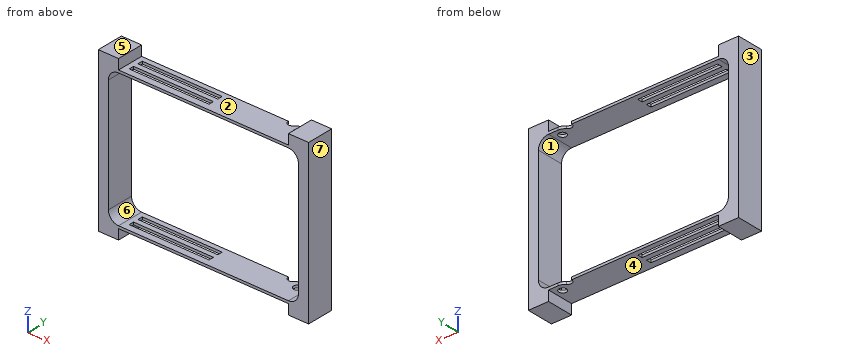
from build123d import *

# Parameters (mm, degrees)
F0_W      = 113
F0_H      = 80
F1_DEPTH  = 15.875
F2_R      = 6
F3_W      = 89
F3_H      = 3
F3_W_2    = 95
F3_R      = 1.5
F4_DEPTH  = 132
F5_W      = 42.9403819144
F5_H      = 7.4070980772
F6_DEPTH  = 1.5
F7_W      = 42.8083911538
F7_H      = 7.2430414148
F8_DEPTH  = 1.5
F9_R      = 2.5
F10_DEPTH = 92
F11_R     = 2.25
F12_DEPTH = 200
F13_R     = 5


with BuildPart() as f1:
    # F0 (on Front) → F1 (new body)
    with BuildSketch(Plane.XZ):
        Polygon((-50.5, 47.5), (-62.5, 47.5), (-62.5, -47.5), (-50.5, -47.5), (-50.5, -41.5), (50.5, -41.5), (50.5, -47.5), (62.5, -47.5), (62.5, 47.5), (50.5, 47.5), (50.5, 41.5), (-50.5, 41.5), align=None)
        Rectangle(F0_W, F0_H, mode=Mode.SUBTRACT)
    extrude(amount=F1_DEPTH)

    # F2
    f2_edges = [f1.edges().sort_by_distance(p)[0] for p in [
        (56.5, -7.9375, 40),
        (56.5, -7.9375, -40),
        (-56.5, -7.9375, -40),
        (-56.5, -7.9375, 40),
    ]]
    fillet(f2_edges, radius=F2_R)

    # F3 (on face) → F4 (cut)
    with BuildSketch(Plane.XY.offset(41.5)):
        with Locations((-3, -4.5)):
            Rectangle(F3_W, F3_H)
        with Locations((0, -10.5)):
            Rectangle(F3_W_2, F3_H)
        with Locations((46, -4.5)):
            Circle(F3_R)
    extrude(amount=-F4_DEPTH, mode=Mode.SUBTRACT)

    # F5 (on face) → F6 (join)
    with BuildSketch(Plane.XY.offset(41.5)):
        with Locations((21.4701909572, -3.7035490386)):
            Rectangle(F5_W, F5_H)
        Polygon((42.9403819144, -7.4070980772), (0, -7.4070980772), (0, -14.1382440925), (49.1435937583, -14.1382440925), (49.1435937583, -7.4070980772), align=None)
    extrude(amount=-F6_DEPTH)

    # F7 (on face) → F8 (join)
    with BuildSketch(Plane(origin=(0, 0, -41.5), x_dir=(1, 0, 0), z_dir=(0, 0, -1))):
        Polygon((49.0116067231, 15.875), (0, 15.875), (0, 7.2430414148), (42.8083911538, 7.2430414148), (49.0116067231, 7.2430414148), align=None)
        with Locations((21.4041955769, 3.6215207074)):
            Rectangle(F7_W, F7_H)
    extrude(amount=-F8_DEPTH)

    # F9 (on face) → F10 (cut)
    with BuildSketch(Plane.XY.offset(41.5)):
        with Locations((39.25, 0)):
            Circle(F9_R)
    extrude(amount=-F10_DEPTH, mode=Mode.SUBTRACT)

    # F11 (on face) → F12 (cut)
    with BuildSketch(Plane.XY.offset(41.5)):
        with Locations((46, -4.5)):
            Circle(F11_R)
    extrude(amount=-F12_DEPTH, mode=Mode.SUBTRACT)

    # F13
    f13_edges = [f1.edges().sort_by_distance(p)[0] for p in [
        (41.75, 0, 40.75),
        (41.75, 0, -40.75),
    ]]
    fillet(f13_edges, radius=F13_R)


solid = f1.part
The model under review builds one solid part; all positions refer to its coordinate system, in mm. Face numbers are marked on the shaded views. A direction names the side the tool comes from. Round coordinates to 2 decimals unless told otherwise and drop trailing zeros. Order: outer loops, then holes, each group sorted by start corner. A loop starts at its lowest first (then second) coordinate and runs counter-clockwise, first axis right, second up. Notation, with made-up numbers: (11, 54.5) -> (22, 54.5) arc R18 ccw to (22, 65.5) -> close; hole circle Ø1 at (-15.75, 43). An arc over 180 degrees is marked (long way). Return JSON: item names as keys, results as strings.
1. Take a section at A-A (z = 29.5). Write out the cut boundary in (x, y) (3 decimals).
Answer block:
{"outline": "(-62.5, -15.875) -> (-56.5, -15.875) -> (-56.5, 0) -> (-62.5, 0) -> close; (56.5, -15.875) -> (62.5, -15.875) -> (62.5, 0) -> (56.5, 0) -> close"}
2. For L1, parallel to Z at x = -45, y = -12.5; L2, parallel to X at y = -13.75, z = 15; L3, parallel to Y at x = 46, z = -40.8 (3 decimals), list the stretches that pass through material, from the lowest coordinate up. Write a range as [from, to].
Answer block:
{"L1": "z = [-41.5, -40], [40, 41.5]", "L2": "x = [-62.5, -56.5], [56.5, 62.5]", "L3": "y = [-15.875, -6.75], [-2.25, 0]"}
3. The part is to be moulded in two halves that separate along X. For the marked faces 5, 6 and 7, say which applies: +X half, -X half, draft (parallel to the pull), parting line (faces both ways), or undercut.
Answer block:
{"face 5": "draft", "face 6": "undercut", "face 7": "+X half"}
4. For the marked faces 1, 2, 3 and 4, list the 3-axis set-ups (+Z, -Z, +X, -X, +Y, -Y) from which the entire face can be reached by the end or side of a thin tool; tool diameter is ignored.
Answer block:
{"face 1": "+Y, -Y", "face 2": "+Z, +Y, -Y", "face 3": "+Z, -Z, -X, +Y, -Y", "face 4": "-Z, +Y, -Y"}
5. Take a section at B-B (y = -4.5). State how many separate pieces and enclosed holes the cut face has, then the cut area to 3 significant figures.
Answer block:
{"separate pieces": "4", "enclosed holes": "0", "area": "1,500 mm²"}
6. Insertion check: P1, Ø5, axis at x = 46, y = -9.5, coming from the -Z side; P2, Ø4, axis at x = 23.5, y = -9, coming from the +Z side. Each pin has a flat end and moves straight along its axis. Give the tip position at first contact, or say it passes through.
Answer block:
{"P1": "stops at z = -41.5", "P2": "stops at z = 41.5"}
7. Take a section at C-C (z = -38). Write out the cut boundary in (x, y) (3 decimals).
Answer block:
{"outline": "(-62.5, -15.875) -> (-54.972, -15.875) -> (-54.972, 0) -> (-62.5, 0) -> close; (54.972, -15.875) -> (62.5, -15.875) -> (62.5, 0) -> (54.972, 0) -> close"}
